Source: CAD feature listing. Evaluate the final solid. Frame: model axes, mm. A direction names the side the tool comes from. Round coordinates to 2 decimals unless told otherwise and drop trailing zeros. Write each loop counter-clockwise with the first axis right and the second up, starting at its lowest first coordinate (ties: lowest second). Pieces come first, ordered by that corner, then holes. Notation, with made-up numbers: M 74.5,-2 L 125.5,-2 A33 ccw 125.5,37 Z; hole C 22.25,-8.75 d8. An arc over 180 degrees is marked long. Answer in a Markdown table with one row per item. Add a question column.
Item 1: Material intervals for probe 1 along Y at (x, z) = (36, 33.5); probe 2 along Y at (x, z) = (-23.5, 16.5); probe 3 along Z at (x, y) = (-17.5, 82) (3 decimals), sorted ascending.
Item 2: Mould query, pull axis Z, two halves, no side actions, for faces 1 (the face through (22.95, 83.891, 2.872)), 2 (the face through (49.89, 6.44, -62.55)), 3 (the face through (-18.199, 45, 57)). Classes: released by +Z, released by -Z, zero draft, split by the parting line, or undercut.
Item 3: Set-up query: faces 4 (the face through (22, 78.74, 26)), 5 (the face through (0, 45, 50.8)), 6 (the face through (17.526, 17, -65)), 7 (the face through (18.199, 45, 57)). Return all of +Z, -Z, +X, -X, +Y, -Y with unobstructed straight access to the full face (end or side cutting, diameter ignored); none if empty.
Item 4: Cut plane A-A on x = -14. Give the number of separate pieces and of enclosed holes in the cut face, and give its area (3 significant figures).
Item 5: Cut plane C-C on z = -45. Return loops of the section in (x, y) (3 decimals).
Item 6: Contact query for flat-ended pins moving along their axis: pin 1 (10 mm diameter, centred on x = -21, y = 9.5, fed in from -Z); pin 2 (5 mm diameter, centred on x = 29, y = 52, fed in from +Z); pin 3 (20.5 mm diameter, centred on y = 25.5, z = -63, fed in from -X) (3 decimals); pin 4 (8 mm diameter, centred on y = 17, z = 7, fed in from +X). Output: stop coordinate, or through.
Item 7: Cut plane D-D on y = 39. Return loops of the section in (x, z) (3 decimals).
Autodesk Inventor part; units mm, degrees
ref_plane "YZ Plane" through (0, 0, 0) normal (1, 0, 0) x (0, 1, 0)
ref_plane "XZ Plane" through (0, 0, 0) normal (0, 1, 0) x (-1, 0, 0)
ref_plane "XY Plane" through (0, 0, 0) normal (0, 0, 1) x (1, 0, 0)
sketch "Sketch1" plane through (0, 0, 0) normal (0, 1, 0) x (-1, 0, 0)
  line L0 (-50.8, -63.5) -> (50.8, -63.5)
  line L1 (50.8, -63.5) -> (50.8, 63.5)
  line L2 (50.8, 63.5) -> (-50.8, 63.5)
  line L3 (-50.8, 63.5) -> (-50.8, -63.5)
  line L4 (-50.8, -63.5) -> (50.8, 63.5) construction
  line L5 (50.8, -63.5) -> (-50.8, 63.5) construction
  point P0 (0, 0)
  dimension "d0" = 101.6
  dimension "d1" = 127
extrude "Extrusion1" add sketch "Sketch1" along normal blind 12.7
fillet "Fillet1" radius 3.175 4 edges at (-50.8, 6.35, 63.5) (50.8, 6.35, 63.5) (50.8, 6.35, -63.5) (-50.8, 6.35, -63.5)
sketch "Sketch2" plane through (0, 12.7, 0) normal (0, 1, 0) x (1, 0, 0)
  line L0 (47.625, 63.5) -> (-47.625, 63.5)
  line L1 (-47.625, 63.5) -> (47.625, 63.5)
  line L2 (47.625, 63.5) -> (47.625, 50.8)
  line L3 (47.625, 50.8) -> (-47.625, 50.8)
  line L4 (-47.625, 50.8) -> (-47.625, 63.5)
  line L5 (-47.625, -39.3448) -> (47.625, -39.3448)
  line L6 (47.625, -39.3448) -> (47.625, -60.325)
  line L7 (47.625, -60.325) -> (-47.625, -60.325)
  line L8 (-47.625, -60.325) -> (-47.625, -39.3448)
  point P0 (0, 0)
  dimension "d5" = 12.7
extrude "Extrusion2" add sketch "Sketch2" along normal blind 76.2 contours L2 L3 L4 L0
sketch "Sketch3" plane through (47.625, 12.7, -50.8) normal (1, 0, 0) x (0, 0, -1)
  point P0 (-50.8, -12.7)
sketch "Sketch4" plane through (-47.625, 12.7, -50.8) normal (0, 0, 1) x (1, 0, 0)
  line L0 (0, 0) -> (0, 76.2)
  line L1 (95.25, 0) -> (98.425, 0)
  line L2 (0, 76.2) -> (95.25, 76.2)
  line L3 (95.25, 76.2) -> (95.25, 0)
  line L4 (95.25, 0) -> (0, 0)
  line L5 (0, 0) -> (0, 76.2)
  point P0 (47.625, -12.7)
extrude "Extrusion3" add sketch "Sketch4" along normal blind 76.2
sketch "Sketch5" plane through (47.625, 12.7, -63.5) normal (1, 0, 0) x (0, 0, -1)
  line L0 (0, 76.2) -> (-88.9, 76.2)
  line L1 (0, 0) -> (0, 76.2)
  line L2 (-44.45, 76.2) -> (0, 0)
  line L3 (0, 0) -> (0, 76.2)
  line L4 (0, 76.2) -> (-44.45, 76.2)
  line L5 (0, 0) -> (-88.9, 0)
  line L6 (-88.9, 0) -> (-44.45, 76.2)
  line L7 (-88.9, 76.2) -> (-88.9, 0)
  line L8 (-88.9, 76.2) -> (-44.45, 76.2)
  point P0 (-63.5, -12.7)
extrude "Extrusion4" cut sketch "Sketch5" against normal blind 95.25 contours L1 L2 L0
sketch "Sketch6" plane through (47.625, 12.7, 25.4) normal (1, 0, 0) x (0, 0, -1)
  line L0 (44.45, 76.2) -> (0, 76.2)
  line L1 (44.45, 76.2) -> (31.75, 76.2)
  line L2 (0, 0) -> (88.9, 0)
  line L3 (88.9, 0) -> (76.2, 0)
  line L4 (76.2, 0) -> (31.75, 76.2)
  line L5 (44.45, 76.2) -> (88.9, 0)
  line L6 (44.45, 76.2) -> (88.9, 0)
  line L7 (88.9, 0) -> (76.2, 0)
  line L8 (0, 76.2) -> (0, 0)
  line L9 (0, 76.2) -> (0, 0)
  line L10 (0, 0) -> (76.2, 0)
  line L11 (31.75, 76.2) -> (0, 76.2)
  point P0 (25.4, -12.7)
  dimension "d12" = 12.7
  dimension "d13" = 12.7
extrude "Extrusion5" cut sketch "Sketch6" against normal blind 95.25 contours L4 L2 L8 L0
sketch "Sketch7" plane through (-47.625, 12.7, -63.5) normal (-1, 0, 0) x (0, 0, 1)
  line L0 (44.45, 76.2) -> (57.15, 76.2)
  line L1 (127, -12.7) -> (127, 0)
  line L2 (57.15, 76.2) -> (127, 0)
  line L3 (57.15, 76.2) -> (127, 76.2)
  line L4 (127, 76.2) -> (127, 0)
  line L5 (57.15, 76.2) -> (12.7, 0)
  line L6 (49.7417, 63.5) -> (127, 63.5)
  point P0 (63.5, -12.7)
  dimension "d16" = 12.7
extrude "Extrusion6" add sketch "Sketch7" against normal blind 95.25 contours L3 L4 L6 L2 | L2 L6 L5
fillet "Fillet2" radius 3.175 2 edges at (47.625, 82.55, 63.5) (-47.625, 82.55, 63.5)
sketch "Sketch8" plane through (47.625, 12.7, -63.5) normal (0, 0.5039, -0.8638) x (-1, 0, 0)
  line L0 (0, 79.9133) -> (0, 6.3992)
  line L1 (95.25, 0) -> (0, 0)
  line L2 (0, 6.3992) -> (95.25, 6.3992)
  line L3 (95.25, 6.3992) -> (95.25, 0)
  line L4 (95.25, 0) -> (0, 0)
  line L5 (0, 0) -> (0, 6.3992)
  point P0 (47.625, 21.0258)
extrude "Extrusion7" add sketch "Sketch8" along normal blind 10.16
fillet "Fillet3" radius 3.175 2 edges at (0, 23.3468, -69.0516) (0, 17.8193, -72.276)
sketch "Sketch9" plane through (0, 88.9, 0) normal (0, 1, 0) x (1, 0, 0)
  line L0 (-44.45, -63.5) -> (44.45, -63.5)
  line L1 (0, -63.5) -> (0, 19.05)
  line L2 (47.625, 19.05) -> (-47.625, 19.05)
  arc A0 (-47.625, -60.325) -> (-44.45, -63.5) centre (-44.45, -60.325) ccw
  circle A1 centre (-22.225, -20.6375) radius 17.78
  circle A2 centre (22.225, -20.6375) radius 17.78
  line L3 (-18.1992, -63.5) -> (-18.1992, -37.9557)
  line L4 (-26.2508, -37.9557) -> (-26.2508, -63.5)
  line L5 (18.1992, -37.9557) -> (18.1992, -63.5)
  line L6 (26.2508, -37.9557) -> (26.2508, -63.5)
  point P0 (0, 0)
  dimension "d23" = 35.56
  dimension "d24" = 35.56
  dimension "d25" = 8.0516
extrude "Extrusion8" cut sketch "Sketch9" against normal blind 10.16
sketch "Sketch10" plane through (-44.45, 76.2, 63.5) normal (0, 0, 1) x (1, 0, 0)
  line L0 (92.075, 0) -> (-3.175, 0)
  line L1 (44.45, 0) -> (44.45, -63.5)
  line L2 (92.075, -63.5) -> (-3.175, -63.5)
  line L3 (62.6492, 2.54) -> (62.6492, 12.7)
  line L4 (62.6492, 2.54) -> (62.6492, -63.5)
  line L5 (26.2508, 2.54) -> (18.1992, 2.54)
  line L6 (26.2508, 2.54) -> (26.2508, -63.5)
  point P0 (44.45, -76.2)
  point P1 (62.6492, 0)
  point P2 (26.2508, 0)
extrude "Extrusion9" add sketch "Sketch10" against normal blind 12.7
sketch "Sketch11" plane through (-47.625, 12.7, -63.5) normal (0, -0.8638, -0.5039) x (1, 0, 0)
  line L0 (95.25, -6.985) -> (0, -6.985)
  line L1 (47.625, -6.985) -> (47.625, 0)
  line L2 (95.25, 0) -> (0, 0)
  line L3 (47.625, -6.985) -> (30.101, -6.985)
  line L4 (30.101, -6.985) -> (30.101, 0)
  line L5 (47.625, -6.985) -> (65.151, -6.985)
  line L6 (65.151, -6.985) -> (65.151, 0)
  line L7 (47.625, 0) -> (30.101, 0)
  point P0 (47.625, 61.2491)
  dimension "d30" = 17.526
extrude "Extrusion10" cut sketch "Sketch11" against normal blind 25.4
properties part number "PhoneStand"
Results below:
| question | item | result |
|---|---|---|
| 1 | probe 1 | 0 to 12.7, 76.2 to 88.9 |
| 1 | probe 2 | 0 to 12.7, 76.2 to 78.74 |
| 1 | probe 3 | -23.075 to 3.497, 37.778 to 63.5 |
| 2 | face 1 | undercut |
| 2 | face 2 | released by -Z |
| 2 | face 3 | zero draft |
| 3 | face 4 | +Y |
| 3 | face 5 | +X, -X |
| 3 | face 6 | none |
| 3 | face 7 | +Z, +X |
| 4 | separate pieces | 2 |
| 4 | enclosed holes | 1 |
| 4 | area | 4,020 mm2 |
| 5 | outline | M -50.8,0 L 50.8,0 L 50.8,12.7 L -50.8,12.7 Z; M -47.625,22.643 L 47.625,22.643 L 47.625,44.414 L -47.625,44.414 Z |
| 6 | pin 1 | z = -66.59 |
| 6 | pin 2 | z = -26.42 |
| 6 | pin 3 | x = -47.625 |
| 6 | pin 4 | through |
| 7 | outline | M -47.625,-48.158 L 47.625,-48.158 L 47.625,-35.458 L -47.625,-35.458 Z; M -18.199,50.8 L 18.199,50.8 L 18.199,63.5 L -18.199,63.5 Z |
